Verification items for the finished model (mm, model axes). A direction names the side the tool comes from. Give positions to 0.01 mm unless a question says otherwise; leave off trailing zeros. Order: outer loops, then holes, each group sorted by start corner. A loop starts at its lowest first (then second) coordinate and runs counter-clockwise, first axis right, second up.
from build123d import *

# Parameters (mm, degrees)
SKETCH_1_W           = 63.4
SKETCH_1_H           = 63.4
EXTRUDE_1_DEPTH      = 22
SKETCH_2_W           = 50
SKETCH_2_H           = 50
CUT_EXTRUDE_1_DEPTH  = 10
SKETCH_3_W           = 54
SKETCH_3_H           = 54
CUT_EXTRUDE_2_DEPTH  = 12
SKETCH_4_W           = 6
SKETCH_4_H           = 54
CUT_EXTRUDE_3_DEPTH  = 2
SKETCH_5_W           = 6
SKETCH_5_H           = 56
CUT_EXTRUDE_4_DEPTH  = 2
SKETCH_6_W           = 6
SKETCH_6_H           = 56
CUT_EXTRUDE_5_DEPTH  = 2
SKETCH_8_W           = 6
SKETCH_8_H           = 58
CUT_EXTRUDE_9_DEPTH  = 2
CUT_EXTRUDE_11_REACH = 4.7
SKETCH_9_W           = 3.5
SKETCH_9_H           = 3.5
SKETCH_10_R          = 2
CUT_EXTRUDE_12_DEPTH = 2
CUT_EXTRUDE_13_REACH = 63.4
SKETCH_11_R          = 1.1
SKETCH_12_R          = 2
CUT_EXTRUDE_14_DEPTH = 2
CUT_EXTRUDE_15_REACH = 65.4
SKETCH_13_R          = 1.1
SKETCH_14_R          = 2
CUT_EXTRUDE_16_DEPTH = 2
CUT_EXTRUDE_17_REACH = 63.4
SKETCH_15_R          = 1.1
SKETCH_16_R          = 2
CUT_EXTRUDE_18_DEPTH = 2
CUT_EXTRUDE_19_REACH = 63.4
SKETCH_17_R          = 1.1
FILLET_1_R           = 2
FILLET_2_R           = 2
FILLET_3_R           = 2
FILLET_4_R           = 2


with BuildPart() as part:
    # 草图1 → 凸台-拉伸1 (new body)
    with BuildSketch(Plane(origin=(0, 0, 0), x_dir=(0, 0, -1), z_dir=(1, 0, 0))):
        Rectangle(SKETCH_1_W, SKETCH_1_H)
    extrude(amount=EXTRUDE_1_DEPTH)

    # 草图2 → 切除-拉伸1 (cut)
    with BuildSketch(Plane(origin=(22, 0, 0), x_dir=(0, 0, -1), z_dir=(1, 0, 0))):
        Rectangle(SKETCH_2_W, SKETCH_2_H)
    extrude(amount=-CUT_EXTRUDE_1_DEPTH, mode=Mode.SUBTRACT)

    # 草图3 → 切除-拉伸2 (cut)
    with BuildSketch(Plane.ZY):
        Rectangle(SKETCH_3_W, SKETCH_3_H)
    extrude(amount=-CUT_EXTRUDE_2_DEPTH, mode=Mode.SUBTRACT)

    # 草图4 → 切除-拉伸3 (cut)
    with BuildSketch(Plane(origin=(0, 27, 0), x_dir=(-1, 0, 0), z_dir=(0, -1, 0))):
        with Locations((-9, 0)):
            Rectangle(SKETCH_4_W, SKETCH_4_H)
    extrude(amount=-CUT_EXTRUDE_3_DEPTH, mode=Mode.SUBTRACT)

    # 草图5 → 切除-拉伸4 (cut)
    with BuildSketch(Plane.XY.offset(-27)):
        with Locations((9, 1)):
            Rectangle(SKETCH_5_W, SKETCH_5_H)
    extrude(amount=-CUT_EXTRUDE_4_DEPTH, mode=Mode.SUBTRACT)

    # 草图6 → 切除-拉伸5 (cut)
    with BuildSketch(Plane(origin=(0, -27, 0), x_dir=(1, 0, 0), z_dir=(0, 1, 0))):
        with Locations((9, 1)):
            Rectangle(SKETCH_6_W, SKETCH_6_H)
    extrude(amount=-CUT_EXTRUDE_5_DEPTH, mode=Mode.SUBTRACT)

    # 草图8 → 切除-拉伸9 (cut)
    with BuildSketch(Plane(origin=(0, 0, 27), x_dir=(-1, 0, 0), z_dir=(0, 0, -1))):
        with Locations((-9, 0)):
            Rectangle(SKETCH_8_W, SKETCH_8_H)
    extrude(amount=-CUT_EXTRUDE_9_DEPTH, mode=Mode.SUBTRACT)

    # 草图9 → 切除-拉伸11 (cut, up to next)
    with BuildSketch(Plane(origin=(0, 29, 0), x_dir=(-1, 0, 0), z_dir=(0, -1, 0)), mode=Mode.PRIVATE) as cut_extrude_11_sk1:
        with Locations((-9, -27.25)):
            Rectangle(SKETCH_9_W, SKETCH_9_H)
    cut_extrude_11_tool1 = extrude(cut_extrude_11_sk1.sketch, amount=-CUT_EXTRUDE_11_REACH, mode=Mode.PRIVATE) & part.part
    add(cut_extrude_11_tool1.solids().sort_by_distance((9, 29, 27.25))[0], mode=Mode.SUBTRACT)

    # 草图10 → 切除-拉伸12 (cut)
    with BuildSketch(Plane(origin=(0, 0, -31.7), x_dir=(-1, 0, 0), z_dir=(0, 0, -1))):
        with Locations((-3, 0)):
            Circle(SKETCH_10_R)
    extrude(amount=-CUT_EXTRUDE_12_DEPTH, mode=Mode.SUBTRACT)

    # 草图11 → 切除-拉伸13 (cut, up to next)
    with BuildSketch(Plane(origin=(0, 0, -29.7), x_dir=(-1, 0, 0), z_dir=(0, 0, -1)), mode=Mode.PRIVATE) as cut_extrude_13_sk1:
        with Locations((-3, 0)):
            Circle(SKETCH_11_R)
    cut_extrude_13_tool1 = extrude(cut_extrude_13_sk1.sketch, amount=-CUT_EXTRUDE_13_REACH, mode=Mode.PRIVATE) & part.part
    add(cut_extrude_13_tool1.solids().sort_by_distance((3, 0, -29.7))[0], mode=Mode.SUBTRACT)

    # 草图12 → 切除-拉伸14 (cut)
    with BuildSketch(Plane.XY.offset(31.7)):
        with Locations((3, 0)):
            Circle(SKETCH_12_R)
    extrude(amount=-CUT_EXTRUDE_14_DEPTH, mode=Mode.SUBTRACT)

    # 草图13 → 切除-拉伸15 (cut, up to next)
    with BuildSketch(Plane.XY.offset(31.7), mode=Mode.PRIVATE) as cut_extrude_15_sk1:
        with Locations((3, 0)):
            Circle(SKETCH_13_R)
    cut_extrude_15_tool1 = extrude(cut_extrude_15_sk1.sketch, amount=-CUT_EXTRUDE_15_REACH, mode=Mode.PRIVATE) & part.part
    add(cut_extrude_15_tool1.solids().sort_by_distance((3, 0, 31.7))[0], mode=Mode.SUBTRACT)

    # 草图14 → 切除-拉伸16 (cut)
    with BuildSketch(Plane(origin=(0, -31.7, 0), x_dir=(-1, 0, 0), z_dir=(0, -1, 0))):
        with Locations((-3, 0)):
            Circle(SKETCH_14_R)
    extrude(amount=-CUT_EXTRUDE_16_DEPTH, mode=Mode.SUBTRACT)

    # 草图15 → 切除-拉伸17 (cut, up to next)
    with BuildSketch(Plane(origin=(0, -29.7, 0), x_dir=(-1, 0, 0), z_dir=(0, -1, 0)), mode=Mode.PRIVATE) as cut_extrude_17_sk1:
        with Locations((-3, 0)):
            Circle(SKETCH_15_R)
    cut_extrude_17_tool1 = extrude(cut_extrude_17_sk1.sketch, amount=-CUT_EXTRUDE_17_REACH, mode=Mode.PRIVATE) & part.part
    add(cut_extrude_17_tool1.solids().sort_by_distance((3, -29.7, 0))[0], mode=Mode.SUBTRACT)

    # 草图16 → 切除-拉伸18 (cut)
    with BuildSketch(Plane(origin=(0, 31.7, 0), x_dir=(1, 0, 0), z_dir=(0, 1, 0))):
        with Locations((3, 0)):
            Circle(SKETCH_16_R)
    extrude(amount=-CUT_EXTRUDE_18_DEPTH, mode=Mode.SUBTRACT)

    # 草图17 → 切除-拉伸19 (cut, up to next)
    with BuildSketch(Plane(origin=(0, 29.7, 0), x_dir=(1, 0, 0), z_dir=(0, 1, 0)), mode=Mode.PRIVATE) as cut_extrude_19_sk1:
        with Locations((3, 0)):
            Circle(SKETCH_17_R)
    cut_extrude_19_tool1 = extrude(cut_extrude_19_sk1.sketch, amount=-CUT_EXTRUDE_19_REACH, mode=Mode.PRIVATE) & part.part
    add(cut_extrude_19_tool1.solids().sort_by_distance((3, 29.7, 0))[0], mode=Mode.SUBTRACT)

    # 圆角1
    fillet_1_edges = [part.edges().sort_by_distance(p)[0] for p in [
        (9, -29, -29),
        (9, -29, 29),
        (9, 29, -29),
    ]]
    fillet(fillet_1_edges, radius=FILLET_1_R)

    # 圆角2
    fillet_2_edges = [part.edges().sort_by_distance(p)[0] for p in [
        (17, 25, -25),
        (17, -25, -25),
        (17, -25, 25),
        (17, 25, 25),
    ]]
    fillet(fillet_2_edges, radius=FILLET_2_R)

    # 圆角3
    fillet_3_edges = [part.edges().sort_by_distance(p)[0] for p in [
        (3, 27, -27),
        (3, 27, 27),
        (3, -27, -27),
        (3, -27, 27),
    ]]
    fillet(fillet_3_edges, radius=FILLET_3_R)

    # 圆角4
    fillet_4_edges = [part.edges().sort_by_distance(p)[0] for p in [
        (11, -31.7, -31.7),
        (11, -31.7, 31.7),
        (11, 31.7, 31.7),
        (11, 31.7, -31.7),
    ]]
    fillet(fillet_4_edges, radius=FILLET_4_R)


solid = part.part
(1) Release check for a two-part mould opening along Z. For faces 1 (the cylindrical face through (11.15, -31.13, -31.1)), 2 (the flat face through (0, 0, 29)), 3 (the flat face through (17, -25, 0)) record: pulls with the +Z half, pulls with the -Z half, needs draft (parallel to the pull), parting line crosses it, or undercut.
Solved:
face 1: pulls with the -Z half
face 2: needs draft
face 3: undercut
(2) Set-up check for faces 4 (the cylindrical face through (3.04, -26.4, -26.43)), 5 (the flat face through (9, -29, 0)), 6 (the cylindrical face through (16.93, 24.4, -24.43)), 7 (the flat face through (4, -1, 29.7)), 8 (the flat face through (7.25, 30, 27)): record each of +Z, -Z, +X, -X, +Y, -Y from which the full face is reachable in a straight line by a thin tool's end or side.
Solved:
face 4: -X
face 5: none
face 6: +X, -X
face 7: +Z
face 8: +Y
(3) Section check C-C, the plane y = 0. Give the number of separate pieces and of enclosed holes in the cut face, then the cut area to 3 significant figures.
Solved:
separate pieces: 4
enclosed holes: 0
area: 195 mm2
(4) Section check D-D, the plane x = 14.5. Enter the section's corners in (y, z).
Solved:
outline: (-31.7, -29.7) arc R2 ccw to (-29.7, -31.7) - (29.7, -31.7) arc R2 ccw to (31.7, -29.7) - (31.7, 29.7) arc R2 ccw to (29.7, 31.7) - (-29.7, 31.7) arc R2 ccw to (-31.7, 29.7) - close; hole (-25, -23) arc R2 ccw to (-23, -25) - (23, -25) arc R2 ccw to (25, -23) - (25, 23) arc R2 ccw to (23, 25) - (-23, 25) arc R2 ccw to (-25, 23) - close
(5) Scan lines: line 1 (Z direction, x = 8.75, y = -8); line 2 (Y direction, x = 13, z = 0.5); line 3 (Z direction, x = 3, y = -28.3). Record each from-to range of solid material in increasing order.
Solved:
line 1: z = -31.7 to -29, 29 to 31.7
line 2: y = -31.7 to -25, 25 to 31.7
line 3: z = -31.7 to -1.1, 1.1 to 31.7
(6) Section check A-A, the plane y = 11. Enter the section's corners in (x, z), then the cut area to 3 significant figures.
Solved:
outline: (0, -31.7) - (22, -31.7) - (22, -25) - (12, -25) - (12, -29) - (6, -29) - (6, -27) - (0, -27) - close; (0, 27) - (6, 27) - (6, 29) - (12, 29) - (12, 25) - (22, 25) - (22, 31.7) - (0, 31.7) - close
area: 223 mm2
(7) Go/stop test with flat-tipped pins: pin 1 (1 mm diameter, centred on y = 23, z = -20, fed in from +X); pin 2 (2 mm diameter, centred on x = 2.5, z = -0.5, fed in from -Y); pin 3 (3.5 mm diameter, centred on x = 3, y = 0, fed in from -Z); pin 4 (1.2 mm diameter, centred on x = 2.5, y = -1, fed in from +Z). Record where each tip stops, or that it passes through.
Solved:
pin 1: passes through
pin 2: stops at y = -29.7
pin 3: stops at z = -29.7
pin 4: stops at z = 29.7
